Here's the drawing with two shaded views (mm, measured from the low corner). I have some questions. A direction names the side the tool comes from. Give positions to 0.01 mm unless a question says otherwise; leave off trailing zeros. Answer as a JSON object with one key per item and string values. Group by question number.
Item 1: Will these pins go through, and if not, where does the flat tip stop? pin 1 (2 mm diameter, centred on x = 7.5, z = 10, fed in from -Y); pin 2 (1 mm diameter, centred on x = 4.5, y = 1, fed in from -Z); pin 3 (3 mm diameter, centred on y = 6.5, z = 14, fed in from +X) (1 decimal).
Item 2: Thinking about a two-plate mould opening in Y: for the marked faces 1, 2 and 3, which applies, pulls with the +Y half, pulls with the -Y half, needs draft (parallel to the pull), parting line crosses it, or undercut?
Item 3: Please list where these lines run through material, in increasing order: L1, parallel to Z at x = 7.5, y = 5.5; L2, parallel to X at y = 3.75, z = 16 (1 decimal); L3, parallel to Z at x = 3, y = 3.5.
Item 4: Which directions (+Z, -Z, +X, -X, +Y, -Y) give clear straight access to the entire face, cutting with the end or side of a thin tool? Please do the marked faces 4 and 5.
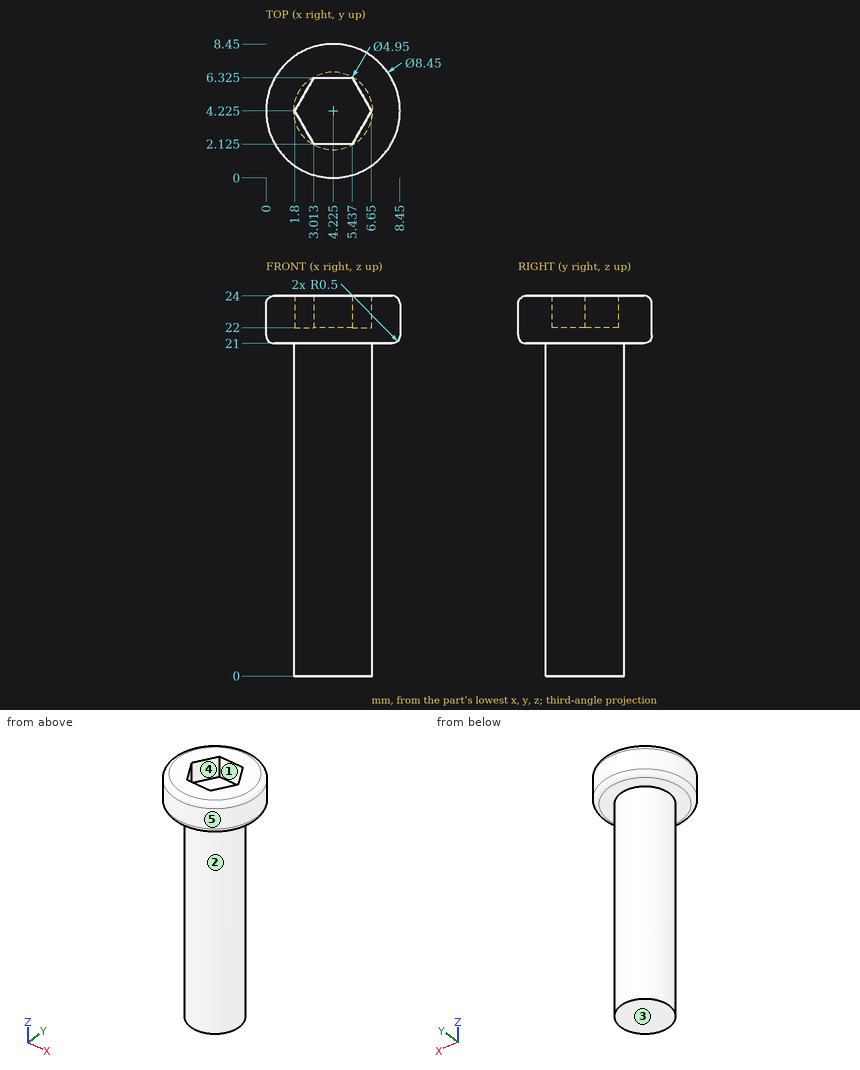
Worked out:
{
 "1": {"pin 1": "stops at y = 3.25", "pin 2": "stops at z = 21", "pin 3": "stops at x = 6.6"},
 "2": {"face 1": "undercut", "face 2": "parting line crosses it", "face 3": "needs draft"},
 "3": {"L1": "z = 21 to 24", "L2": "x = 1.8 to 6.7", "L3": "z = 0 to 22"},
 "4": {"face 4": "+Z", "face 5": "+Z, -Z"}
}
